Design review of the part built by this model. Coordinates are the model's own, in mm. Face numbers are marked on the shaded views. Coordinates: 2 decimals unless noted, no trailing zeros. Write each loop counter-clockwise with the first axis right and the second up, starting at its lowest first coordinate (ties: lowest second). Pieces come first, ordered by that corner, then holes. Notation, with made-up numbers: M -8,36 L 20,36 A8 ccw 20,42 Z; hole C 17,14 d5. An arc over 180 degrees is marked long. One line per question, with ' | ' between items.
from build123d import *

# Parameters (mm, degrees)
SKETCH_1_W      = 185
SKETCH_1_H      = 99
EXTRUDE_1_DEPTH = 5
EXTRUDE_2_DEPTH = 8
EXTRUDE_3_DEPTH = 2
SKETCH_4_W      = 5
SKETCH_4_H      = 99
EXTRUDE_4_DEPTH = 20
SKETCH_5_W      = 5
SKETCH_5_H      = 5
EXTRUDE_5_DEPTH = 40


with BuildPart() as part:
    # Sketch 1 → Extrude 1 (new body)
    with BuildSketch(Plane(origin=(0, 0, 0), x_dir=(1, 0, 0), z_dir=(0, 1, 0))):
        with Locations((9.615231102, 5.409140969)):
            Rectangle(SKETCH_1_W, SKETCH_1_H)
    extrude(amount=EXTRUDE_1_DEPTH)

    # Sketch 3 → Extrude 2 (add)
    with BuildSketch(Plane(origin=(0, 0, 0), x_dir=(1, 0, 0), z_dir=(0, 1, 0))):
        Polygon((-77.884768898, -39.090859031), (-77.884768898, 49.909140969), (-77.884768898, 54.909140969), (-82.884768898, 54.909140969), (-82.884768898, -39.090859031), align=None)
        Polygon((-77.884768898, 54.909140969), (-77.884768898, 49.909140969), (97.115231102, 49.909140969), (97.115231102, -39.090859031), (-77.884768898, -39.090859031), (-82.884768898, -39.090859031), (-82.884768898, -44.090859031), (102.115231102, -44.090859031), (102.115231102, 54.909140969), align=None)
    extrude(amount=EXTRUDE_2_DEPTH)

    # Sketch 3_3 → Extrude 3 (add)
    with BuildSketch(Plane(origin=(0, 0, 0), x_dir=(1, 0, 0), z_dir=(0, 1, 0))):
        Polygon((-77.884768898, 54.909140969), (-77.884768898, 49.909140969), (97.115231102, 49.909140969), (97.115231102, -39.090859031), (-77.884768898, -39.090859031), (-82.884768898, -39.090859031), (-82.884768898, -44.090859031), (102.115231102, -44.090859031), (102.115231102, 54.909140969), align=None)
        Polygon((-77.884768898, -39.090859031), (-77.884768898, 49.909140969), (-77.884768898, 54.909140969), (-82.884768898, 54.909140969), (-82.884768898, -39.090859031), align=None)
    extrude(amount=-EXTRUDE_3_DEPTH)

    # Sketch 4 → Extrude 4 (add)
    with BuildSketch(Plane(origin=(0, 0, 0), x_dir=(1, 0, 0), z_dir=(0, 1, 0))):
        with Locations((-80.384768898, 5.409140969)):
            Rectangle(SKETCH_4_W, SKETCH_4_H)
    extrude(amount=-EXTRUDE_4_DEPTH)

    # Sketch 5 → Extrude 5 (add)
    with BuildSketch(Plane(origin=(0, 0, 0), x_dir=(1, 0, 0), z_dir=(0, 1, 0))):
        with Locations((-80.384768898, 52.409140969)):
            Rectangle(SKETCH_5_W, SKETCH_5_H)
        with Locations((99.615231102, 52.409140969)):
            Rectangle(SKETCH_5_W, SKETCH_5_H)
        with Locations((99.615231102, -41.590859031)):
            Rectangle(SKETCH_5_W, SKETCH_5_H)
        with Locations((-80.384768898, -41.590859031)):
            Rectangle(SKETCH_5_W, SKETCH_5_H)
    extrude(amount=EXTRUDE_5_DEPTH)


solid = part.part
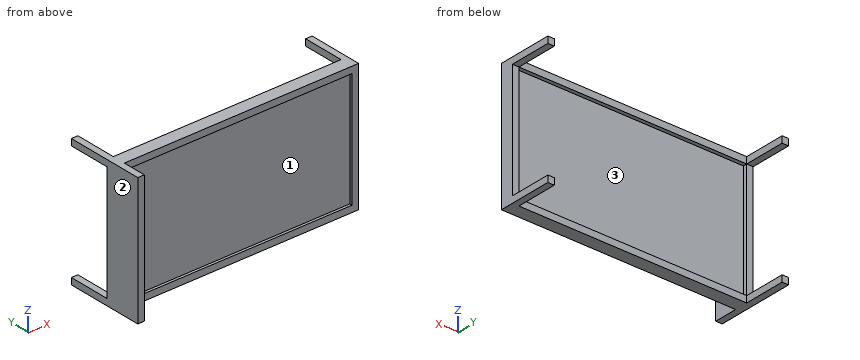
1. To check wall thickness, follow line 1 along Z through (x, y) = (2, 7.5); line 2 along X through (y, z) = (-7, 30); line 3 along Y through (x, z) = (-38.5, -18.5). State the ranges of each line that lie inside material, in increasing order. Write a range as [from, to].
Answer sheet:
line 1: [-54.91, -49.91], [39.09, 44.09] | line 2: [-82.88, -77.88] | line 3: [0, 5]
2. Take a section at D-D (y = -12). Write out the cut boundary in (x, z), then the cut area to 3 significant figures.
Answer sheet:
outline: M -82.88,-54.91 L -77.88,-54.91 L -77.88,44.09 L -82.88,44.09 Z | area: 495 mm^2
3. Insertion check: pin 1 Ø3 at (x, z) = (73.5, -15.5) entering from -Y; pin 2 Ø6 at (y, z) = (-13, -44.5) entering from +X; pin 3 Ø12 at (x, y) = (-32.5, -2.5) entering from -Z; pin 4 Ø4 at (x, z) = (99, 4.5) entering from +Y. Each pin has a flat end and moves straight along its axis. Give the tip position at first contact, or say it passes through.
Answer sheet:
pin 1: y = 0 | pin 2: x = -77.88 | pin 3: z = -54.91 | pin 4: y = 8
4. Draft analysis for pull direction Z (two halves, no side actions). For the marked faces 1, 2 and 3, state which applies: pulls with the +Z half, pulls with the -Z half, needs draft (parallel to the pull), parting line crosses it, or undercut.
Answer sheet:
face 1: undercut | face 2: needs draft | face 3: undercut
5. Take a section at C-C (x = -17.5). Write out the cut boundary in (y, z), then the cut area to 3 significant figures.
Answer sheet:
outline: M -2,-54.91 L 8,-54.91 L 8,-49.91 L 5,-49.91 L 5,39.09 L 8,39.09 L 8,44.09 L -2,44.09 L -2,39.09 L 0,39.09 L 0,-49.91 L -2,-49.91 Z | area: 545 mm^2
6. Take a section at B-B (z = 28.5). Write out the cut boundary in (x, y).
Answer sheet:
outline: M -82.88,-20 L -77.88,-20 L -77.88,0 L 97.12,0 L 97.12,-2 L 102.12,-2 L 102.12,8 L 97.12,8 L 97.12,5 L -77.88,5 L -77.88,8 L -82.88,8 Z
7. Take a section at A-A (y = 23.5). Write out the cut boundary in (x, z).
Answer sheet:
outline: M -82.88,-54.91 L -77.88,-54.91 L -77.88,-49.91 L -82.88,-49.91 Z; M -82.88,39.09 L -77.88,39.09 L -77.88,44.09 L -82.88,44.09 Z; M 97.12,-54.91 L 102.12,-54.91 L 102.12,-49.91 L 97.12,-49.91 Z; M 97.12,39.09 L 102.12,39.09 L 102.12,44.09 L 97.12,44.09 Z
